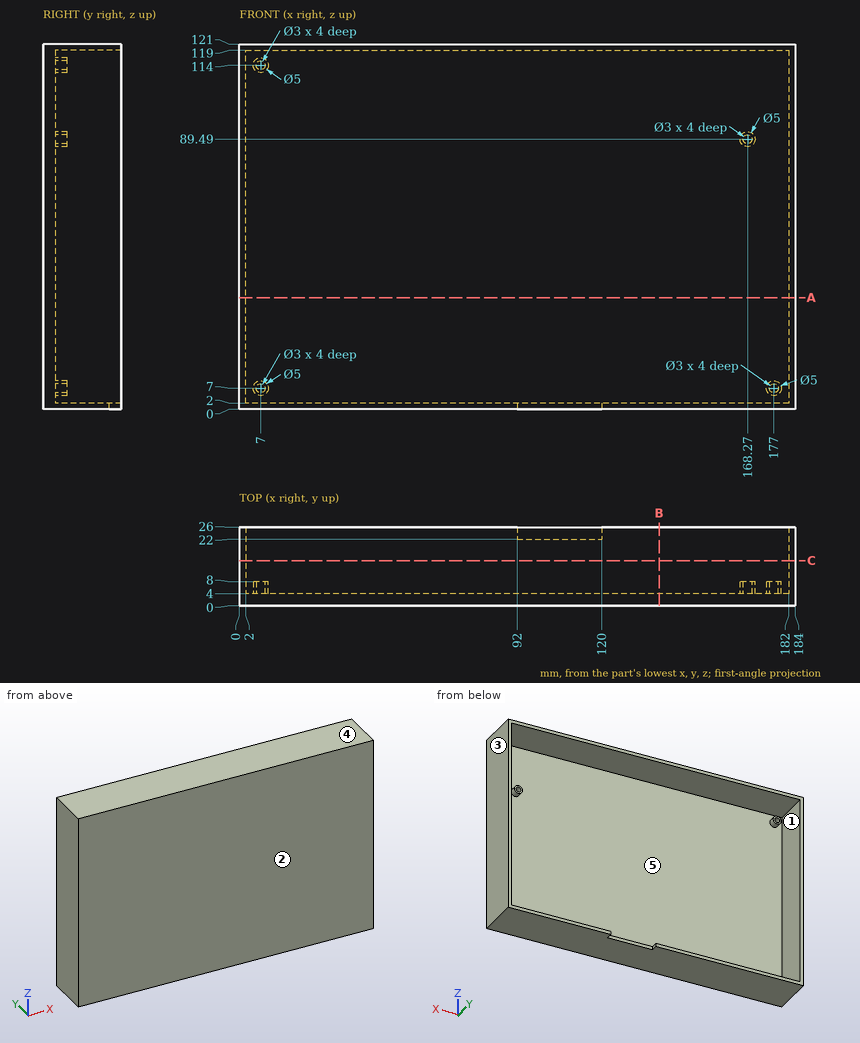
Design review of the part shown in the three views and the two pictorial views. Dimensions are in mm from the part's minimum x, y and z. A direction names the side the tool comes from. Round coordinates to 2 decimals unless told otherwise and drop trailing zeros. Order: outer loops, then holes, each group sorted by start corner. A loop starts at its lowest first (then second) coordinate and runs counter-clockwise, first axis right, second up. Notation, with made-up numbers: (64.5, -23) - (70.5, -23) arc R26 ccw to (70.5, -6) - close; hole circle Ø10 at (0, 82.25). An arc over 180 degrees is marked (long way). One line per question, with ' | ' between items.
Item 1: Machinability: for the marked faces 1 and 2, which of the approach directions +Z, -Z, +X, -X, +Y, -Y give a long, thin tool a straight path to every point of the face, cutting with its end or side? Answer none if there is none.
Checks:
face 1: +Y | face 2: +Z, -Z, +X, -X, -Y
Item 2: Take a section at B-B, the plane x = 139. Write out the cut boundary in (y, z).
Checks:
outline: (0, 0) - (26, 0) - (26, 2) - (4, 2) - (4, 119) - (26, 119) - (26, 121) - (0, 121) - close
Item 3: Take a section at C-C, the plane y = 15. Write out the cut boundary in (x, z).
Checks:
outline: (0, 0) - (184, 0) - (184, 121) - (0, 121) - close; hole (2, 2) - (182, 2) - (182, 119) - (2, 119) - close
Item 4: Draft analysis for pull direction Z (two halves, no side actions). For the marked faces 3, 4 and 5, state which applies: +Z half, -Z half, draft (parallel to the pull), parting line (faces both ways), or undercut.
Checks:
face 3: draft | face 4: +Z half | face 5: undercut
Item 5: Take a section at A-A, the plane z = 37. Write out the cut boundary in (x, y), then the cut area to 3 significant figures.
Checks:
outline: (0, 0) - (184, 0) - (184, 26) - (182, 26) - (182, 4) - (2, 4) - (2, 26) - (0, 26) - close | area: 824 mm²
Item 6: For P1, Ø10, axis at x = 76, z = 37, coming from the +Y side; P2, Ø2.5, axis at x = 6.5, z = 114.5, coming from the +Y side; P3, Ø2, axis at x = 110, z = 0.5, coming from the +Y side, all flat-tipped, find the tip position at first contact; note any pin that passes through.
Checks:
P1: y = 4 | P2: y = 8 | P3: y = 22
Item 7: Wall thickness on line 1 (X direction, y = 6.7, z = 7); line 2 (X direction, y = 5.7, z = 89.49); line 3 (Z direction, x = 168.27, y = 4.95): over which ranges is each line inside the solid? List them lowest first. Write a range as [from, to].
Checks:
line 1: [0, 2], [4.5, 5.5], [8.5, 9.5], [174.5, 175.5], [178.5, 179.5], [182, 184] | line 2: [0, 2], [165.77, 166.77], [169.77, 170.77], [182, 184] | line 3: [0, 2], [86.99, 87.99], [90.99, 91.99], [119, 121]
